```python
from build123d import *

# Parameters (mm, degrees)
SKETCH_1_R          = 3
EXTRUDE_1_DEPTH     = 32
SKETCH_2_R          = 11
SKETCH_2_R_2        = 7
EXTRUDE_4_DEPTH     = 10
SKETCH_2_5_R        = 7
CUT_EXTRUDE_1_DEPTH = 146.263175934


with BuildPart() as part:
    # Sketch 1 → Extrude 1 (new body)
    # profile 1 of 2: a face of its own
    with BuildSketch(Plane.XY):
        with BuildLine():
            ThreePointArc((116.654846444, 16.380681842), (126.563369948, 22.647533894), (114.944745727, 21.079144946))
            Line((114.944745727, 21.079144946), (90, 12))
            Line((90, 12), (0, 12))
            Line((0, 12), (0, 0))
            Line((0, 0), (90, 0))
            Line((90, 0), (90, 6.679111138))
            Line((90, 6.679111138), (116.654846444, 16.380681842))
        make_face()
        with Locations((120.925214223, 20.595413034)):
            Circle(SKETCH_1_R, mode=Mode.SUBTRACT)
    # profile 2 of 2: a face of its own
    with BuildSketch(Plane.XY):
        with BuildLine():
            Line((138.864016281, 29.785047453), (125.195582003, 24.810144227))
            ThreePointArc((125.195582003, 24.810144227), (126.563369948, 22.647533894), (126.90568272, 20.111681123))
            Line((126.90568272, 20.111681123), (140.574116997, 25.086584349))
            Line((140.574116997, 25.086584349), (138.864016281, 29.785047453))
        make_face()
    extrude(amount=EXTRUDE_1_DEPTH)

    # Sketch 2 → Extrude 4 (add)
    with BuildSketch(Plane(origin=(0, 12, 0), x_dir=(1, 0, 0), z_dir=(0, 1, 0))):
        with Locations(Location((38, -16, 0), (0, 0, 270))):
            Circle(SKETCH_2_R)
        with Locations(Location((38, -16, 0), (0, 0, 270))):
            Circle(SKETCH_2_R_2, mode=Mode.SUBTRACT)
    extrude(amount=EXTRUDE_4_DEPTH)

    # Sketch 2_5 → Cut-Extrude 1 (cut, through all)
    with BuildSketch(Plane(origin=(0, 12, 0), x_dir=(1, 0, 0), z_dir=(0, 1, 0))):
        with Locations(Location((38, -16, 0), (0, 0, 270))):
            Circle(SKETCH_2_5_R)
    extrude(amount=-CUT_EXTRUDE_1_DEPTH, mode=Mode.SUBTRACT)


solid = part.part
```
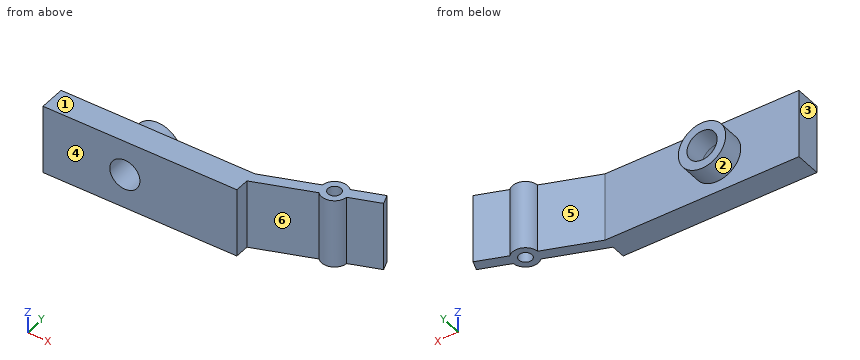
The model under review builds one solid part; all positions refer to its coordinate system, in mm. Face numbers are marked on the shaded views. A direction names the side the tool comes from. Round coordinates to 2 decimals unless told otherwise and drop trailing zeros. Order: outer loops, then holes, each group sorted by start corner. A loop starts at its lowest first (then second) coordinate and runs counter-clockwise, first axis right, second up.
Item 1: Add section D-D, the plane z = 30.5. State the section outline as (x, y) points.
Working result:
outline: (0, 0) - (90, 0) - (90, 6.68) - (116.65, 16.38) arc R6 ccw to (126.91, 20.11) - (140.57, 25.09) - (138.86, 29.79) - (125.2, 24.81) arc R6 ccw to (114.94, 21.08) - (90, 12) - (0, 12) - close; hole circle Ø6 at (120.93, 20.6)
Item 2: For pin 1 (6 mm diameter, centred on x = 41, z = 23.5, fed in from -Y); pin 2 (2 mm diameter, centred on y = 2.5, z = 13.5, fed in from +X); pin 3 (11 mm diameter, centred on x = 38, z = 16, fed in from -Y); pin 4 (5 mm diameter, centred on y = 14.5, z = 18.5, fed in from +X), all flat-tipped, find the tip position at first contact; note any pin that passes through.
Working result:
pin 1: stops at y = 0
pin 2: stops at x = 90
pin 3: passes through
pin 4: stops at x = 125.73
Item 3: To check wall thickness, follow probe 1 along Y at (x, z) = (15, 18); probe 2 along Z at (x, y) = (39, 9.75); probe 3 along Y at (x, z) = (123.5, 5). State the ranges of each line that lie inside material, in increasing order.
Working result:
probe 1: y = 0 to 12
probe 2: z = 0 to 9.07, 22.93 to 32
probe 3: y = 15.18 to 19.06, 22.14 to 26.01
Item 4: Draft analysis for pull direction X (two halves, no side actions). For the marked faces 1, 2 and 3, state which applies: released by +X, released by -X, zero draft, split by the parting line, or undercut.
Working result:
face 1: zero draft
face 2: undercut
face 3: released by -X
Item 5: Add section C-C, the plane y = 4. State the section outline as (x, z) points, and give its area (3 significant figures).
Working result:
outline: (0, 0) - (90, 0) - (90, 32) - (0, 32) - close; hole circle Ø14 at (38, 16)
area: 2,730 mm2
Item 6: Add section A-A, the plane x = 38. State the section outline as (y, z) points.
Working result:
outline: (0, 0) - (12, 0) - (12, 5) - (22, 5) - (22, 9) - (0, 9) - close; (0, 23) - (22, 23) - (22, 27) - (12, 27) - (12, 32) - (0, 32) - close
Item 7: Add section B-B, the plane z = 16. State the section outline as (x, y) points, and give its area (3 significant figures).
Working result:
outline: (0, 0) - (31, 0) - (31, 22) - (27, 22) - (27, 12) - (0, 12) - close; (45, 0) - (90, 0) - (90, 6.68) - (116.65, 16.38) arc R6 ccw to (126.91, 20.11) - (140.57, 25.09) - (138.86, 29.79) - (125.2, 24.81) arc R6 ccw to (114.94, 21.08) - (90, 12) - (49, 12) - (49, 22) - (45, 22) - close; hole circle Ø6 at (120.93, 20.6)
area: 1,280 mm2
Item 8: Machinability: for the marked faces 4, 5 and 6, which of the approach directions +Z, -Z, +X, -X, +Y, -Y give a long, thin tool a straight path to every point of the face, cutting with its end or side? Answer none if there is none.
Working result:
face 4: +Z, -Z, +X, -X, -Y
face 5: +Z, -Z, +Y
face 6: +Z, -Z, -Y
